from build123d import *

# Parameters (mm, degrees)
F0_R     = 15
F1_DEPTH = 7.5
F2_R     = 7.5
F3_DEPTH = 15
F4_R     = 5
F5_DEPTH = 22
F6_R     = 7.5
F7_DEPTH = 15.0010001


with BuildPart() as f1:
    # F0 (on Front) → F1 (new body, symmetric)
    with BuildSketch(Plane.XZ):
        Circle(F0_R)
    extrude(amount=F1_DEPTH, both=True)

    # F2 (on Right) → F3 (join, symmetric)
    with BuildSketch(Plane.YZ):
        Circle(F2_R)
    extrude(amount=F3_DEPTH, both=True)

    # F4 (on Right) → F5 (join, symmetric)
    with BuildSketch(Plane.YZ):
        Circle(F4_R)
    extrude(amount=F5_DEPTH, both=True)

    # F6 (on face) → F7 (cut, through all)
    with BuildSketch(Plane.XZ.offset(7.5)):
        Circle(F6_R)
    extrude(amount=-F7_DEPTH, mode=Mode.SUBTRACT)


solid = f1.part
Input: part model. Units: mm. Frame: model coordinates. A direction names the side the tool comes from. Round coordinates to 2 decimals unless told otherwise and drop trailing zeros. Write each loop counter-clockwise with the first axis right and the second up, starting at its lowest first coordinate (ties: lowest second). Pieces come first, ordered by that corner, then holes.
1) Cut plane B-B (z = -6). Return the cut outline in (x, y), then the cut area to 3 significant figures.
2) Draft query along X for faces 1 (the flat face through (15, 2, -5)), 2 (the cylindrical face through (0, 0, -15)), 3 (the flat face through (-4, -7.5, 7)), 4 (the cylindrical face through (-7.493, -0.105, 0.33)). Return one class per face: pulls with the +X half, pulls with the -X half, needs draft (parallel to the pull), parting line crosses it, or undercut.
3) Cut plane C-C (y = -3). Return the cut outline in (x, z), then the cut area to 3 significant figures.
4) Cut plane A-A (x = 0). Return the cut outline in (y, z).
5) Ray query, L1, parallel to Z at x = 0, y = 3.5; L2, parallel to X at y = 6, z = -5.5; L3, parallel to X at y = 2.5, z = 1. Return the intervals inside material, ascending.
6) Reachability of faces 5 (the cylindrical face through (14.23, 0.16, 7.5)), 6 (the cylindrical face through (-14.2, 0.16, 7.5)), 7 (the cylindrical face through (18.55, -1.08, -4.88)), 8 (the cylindrical face through (-14.2, -0.16, -7.5)), 9 (the cylindrical face through (14.23, -0.16, -7.5)) from +Z, -Z, +X, -X, +Y, -Y: full face, straight path, thin tool, end or side. Return the list, or none.
7) Contact query for flat-ended pins moving along their axis: P1, Ø12, axis at x = 0, z = 0, coming from the -Y side; P2, Ø4, axis at x = -7, y = 4.5, coming from the +Z side; P3, Ø4, axis at y = -1.5, z = -10.5, coming from the +X side; P4, Ø2, axis at x = -2.5, y = -3, coming from the -Z side. Output: stop coordinate, or through.
8) Cut plane D-D (z = 7). Return the cut outline in (x, y).
Geometry says:
1. outline: (-15, -4.5) - (-13.75, -4.5) - (-13.75, -7.5) - (-4.5, -7.5) - (-4.5, 7.5) - (-13.75, 7.5) - (-13.75, 4.5) - (-15, 4.5) - close; (4.5, -7.5) - (13.75, -7.5) - (13.75, -4.5) - (15, -4.5) - (15, 4.5) - (13.75, 4.5) - (13.75, 7.5) - (4.5, 7.5) - close
1. area: 300 mm2
2. face 1: pulls with the +X half
2. face 2: parting line crosses it
2. face 3: needs draft
2. face 4: undercut
3. outline: (-22, -4) - (-15, -4) - (-15, -6.87) - (-13.33, -6.87) arc R15 ccw to (13.33, -6.87) - (15, -6.87) - (15, -4) - (22, -4) - (22, 4) - (15, 4) - (15, 6.87) - (13.33, 6.87) arc R15 ccw to (-13.33, 6.87) - (-15, 6.87) - (-15, 4) - (-22, 4) - close; hole circle Ø15 at (0, 0)
3. area: 657 mm2
4. outline: (-7.5, -15) - (7.5, -15) - (7.5, -7.5) - (-7.5, -7.5) - close; (-7.5, 7.5) - (7.5, 7.5) - (7.5, 15) - (-7.5, 15) - close
5. L1: z = -15 to -7.5, 7.5 to 15
5. L2: x = -13.96 to -5.1, 5.1 to 13.96
5. L3: x = -22 to -7.43, 7.43 to 22
6. face 5: +Z, +X
6. face 6: +Z, -X
6. face 7: +X
6. face 8: -Z, -X
6. face 9: -Z, +X
7. P1: passes through
7. P2: stops at z = 14.14
7. P3: stops at x = 12.36
7. P4: stops at z = -14.92
8. outline: (-15, -2.69) - (-13.27, -2.69) - (-13.27, -7.5) - (-2.69, -7.5) - (-2.69, 7.5) - (-13.27, 7.5) - (-13.27, 2.69) - (-15, 2.69) - close; (2.69, -7.5) - (13.27, -7.5) - (13.27, -2.69) - (15, -2.69) - (15, 2.69) - (13.27, 2.69) - (13.27, 7.5) - (2.69, 7.5) - close
